```python
from build123d import *

# Parameters (mm, degrees)
F0_R        = 2.5
F1_DEPTH    = 3
F3_DEPTH    = 1
F4_T1_DEPTH = 1


# Not quite as in the source:
# - a fillet or chamfer that OpenCascade refuses, or shapes differently, is made with other operations: its cross-section is extruded or revolved along the edge and cut away or added


with BuildPart() as f1:
    # F0 (on Top) → F1 (new body)
    with BuildSketch(Plane.XY):
        with BuildLine():
            Line((42.1995138221, 67.0275468757), (33.4926469464, 67.1294207869))
            ThreePointArc((33.4926469464, 67.1294207869), (32.7404851321, 62.3046461892), (30.658157874, 57.8878475177))
            ThreePointArc((30.658157874, 57.8878475177), (27.294204133, 42.9798709067), (13.9152540739, 50.3668626301))
            ThreePointArc((13.9152540739, 50.3668626301), (12.375918121, 50.6607466073), (10.86986377, 51.0940170307))
            Line((10.86986377, 51.0940170307), (8.0824060906, 42.844775322))
            ThreePointArc((8.0824060906, 42.844775322), (12.4386086282, 40.6384895823), (15.9957592753, 37.2932128243))
            ThreePointArc((15.9957592753, 37.2932128243), (29.1345687017, 29.4870845738), (17.9747991522, 19.0456529188))
            ThreePointArc((17.9747991522, 19.0456529188), (17.2196179112, 17.6724725733), (16.3421568627, 16.3740176929))
            Line((16.3421568627, 16.3740176929), (23.3262801503, 11.1738320243))
            ThreePointArc((23.3262801503, 11.1738320243), (26.7707231948, 14.6350470461), (31.0514904559, 16.9843509793))
            ThreePointArc((31.0514904559, 16.9843509793), (42.5356749941, 27.0678750109), (49.017508165, 13.2277236335))
            ThreePointArc((49.017508165, 13.2277236335), (50.0901164433, 12.0851675302), (51.0538700425, 10.8494078578))
            Line((51.0538700425, 10.8494078578), (58.1577532953, 15.8847580755))
            ThreePointArc((58.1577532953, 15.8847580755), (55.9303336315, 20.230192341), (55.0188426496, 25.0274187796))
            ThreePointArc((55.0188426496, 25.0274187796), (48.977649601, 39.065507608), (64.1434123595, 40.9532553024))
            ThreePointArc((64.1434123595, 40.9532553024), (65.5615019731, 41.620297142), (67.0345955027, 42.1550105429))
            Line((67.0345955027, 42.1550105429), (64.4409135174, 50.4672137913))
            ThreePointArc((64.4409135174, 50.4672137913), (59.6198494134, 49.6916248415), (54.7757497452, 50.307169899))
            ThreePointArc((54.7757497452, 50.307169899), (39.5579025703, 48.8996619005), (42.4490262494, 63.9065055152))
            ThreePointArc((42.4490262494, 63.9065055152), (42.2528455514, 65.4613161473), (42.1995138221, 67.0275468757))
        make_face()
        with Locations((37.5, 37.5)):
            Circle(F0_R, mode=Mode.SUBTRACT)
    extrude(amount=F1_DEPTH)

    # F2 (on face) → F3 (cut)
    with BuildSketch(Plane.XY.offset(3)):
        Polygon((40.25, 67.1147092408), (34.75, 67.1147092408), (40.25, 67.0503569865), align=None)
        with BuildLine():
            Line((31.7569283434, 42.2575582148), (28.1635644564, 43.4251129174))
            ThreePointArc((28.1635644564, 43.4251129174), (20.4254111601, 42.6084822131), (14.6451171229, 47.8175227185))
            Line((14.6451171229, 47.8175227185), (10.2457371637, 49.2469679185))
            Line((10.2457371637, 49.2469679185), (8.4849410638, 44.0360430191))
            Line((8.4849410638, 44.0360430191), (30.0573348743, 37.0267473751))
            Line((30.0573348743, 37.0267473751), (31.7569283434, 42.2575582148))
        make_face()
        with BuildLine():
            Line((31.2005865164, 33.5081806175), (28.9797655003, 30.4514827223))
            ThreePointArc((28.9797655003, 30.4514827223), (27.3652065793, 22.8397088401), (20.6249055731, 18.9520045705))
            Line((20.6249055731, 18.9520045705), (17.9059392288, 15.2096684519))
            Line((17.9059392288, 15.2096684519), (22.3177073919, 11.9247874969))
            Line((22.3177073919, 11.9247874969), (35.6501799855, 30.2753617299))
            Line((35.6501799855, 30.2753617299), (31.2005865164, 33.5081806175))
        make_face()
        with BuildLine():
            Line((52.6444673021, 11.9768495643), (57.1318860772, 15.1576063845))
            Line((57.1318860772, 15.1576063845), (43.7994134836, 33.5081806175))
            Line((43.7994134836, 33.5081806175), (39.3498200145, 30.2753617299))
            Line((39.3498200145, 30.2753617299), (41.5706410307, 27.2186638347))
            ThreePointArc((41.5706410307, 27.2186638347), (48.3109420369, 23.3309595651), (49.9255009579, 15.7191856828))
            Line((49.9255009579, 15.7191856828), (52.6444673021, 11.9768495643))
        make_face()
        with BuildLine():
            Line((66.4538563054, 44.0161570789), (64.8154654671, 49.2668538587))
            Line((64.8154654671, 49.2668538587), (43.2430716566, 42.2575582148))
            Line((43.2430716566, 42.2575582148), (44.9426651257, 37.0267473751))
            Line((44.9426651257, 37.0267473751), (48.5360290127, 38.1943020778))
            ThreePointArc((48.5360290127, 38.1943020778), (54.3163230499, 43.4033425831), (62.0544763461, 42.5867118789))
            Line((62.0544763461, 42.5867118789), (66.4538563054, 44.0161570789))
        make_face()
        with BuildLine():
            Line((34.75, 44.4321520627), (37.5, 44.4321520627))
            Line((37.5, 44.4321520627), (40.25, 44.4321520627))
            Line((40.25, 44.4321520627), (40.25, 48.2104384478))
            ThreePointArc((40.25, 48.2104384478), (37.0821171737, 55.3175067985), (40.25, 62.4245751493))
            Line((40.25, 62.4245751493), (40.25, 67.0503569865))
            Line((40.25, 67.0503569865), (34.75, 67.1147092408))
            Line((34.75, 67.1147092408), (34.75, 44.4321520627))
        make_face()
    extrude(amount=-F3_DEPTH, mode=Mode.SUBTRACT)

    # F4: fillet of radius 3 on 10 edges, made by hand

    # F4_s2 → F4_t1 (join)
    with BuildSketch(Plane.XY.offset(2)):
        with BuildLine():
            ThreePointArc((37.25, 44.4321520627), (39.3713203436, 45.3108317191), (40.25, 47.4321520627))
            Line((40.25, 47.4321520627), (40.25, 44.4321520627))
            Line((40.25, 44.4321520627), (37.25, 44.4321520627))
        make_face()
        with BuildLine():
            ThreePointArc((34.75, 47.4321520627), (35.6286796564, 45.3108317191), (37.75, 44.4321520627))
            Line((37.75, 44.4321520627), (34.75, 44.4321520627))
            Line((34.75, 44.4321520627), (34.75, 47.4321520627))
        make_face()
        with BuildLine():
            ThreePointArc((30.8298773603, 39.4043886659), (30.6497273839, 41.6934111482), (28.9037587945, 43.1846091979))
            Line((28.9037587945, 43.1846091979), (31.7569283434, 42.2575582148))
            Line((31.7569283434, 42.2575582148), (30.8298773603, 39.4043886659))
        make_face()
        with BuildLine():
            ThreePointArc((27.2041653254, 37.9537983583), (29.4931878078, 38.1339483346), (30.9843858575, 39.879916924))
            Line((30.9843858575, 39.879916924), (30.0573348743, 37.0267473751))
            Line((30.0573348743, 37.0267473751), (27.2041653254, 37.9537983583))
        make_face()
        with BuildLine():
            ThreePointArc((33.6276374995, 31.7448248606), (31.3949783475, 32.2808388993), (29.4372307595, 31.0811296344))
            Line((29.4372307595, 31.0811296344), (31.2005865164, 33.5081806175))
            Line((31.2005865164, 33.5081806175), (33.6276374995, 31.7448248606))
        make_face()
        with BuildLine():
            ThreePointArc((33.8868242286, 27.8483107468), (34.4228382672, 30.0809698988), (33.2231290023, 32.0387174868))
            Line((33.2231290023, 32.0387174868), (35.6501799855, 30.2753617299))
            Line((35.6501799855, 30.2753617299), (33.8868242286, 27.8483107468))
        make_face()
        with BuildLine():
            ThreePointArc((41.1131757714, 27.8483107468), (40.5771617328, 30.0809698988), (41.7768709977, 32.0387174868))
            Line((41.7768709977, 32.0387174868), (39.3498200145, 30.2753617299))
            Line((39.3498200145, 30.2753617299), (41.1131757714, 27.8483107468))
        make_face()
        with BuildLine():
            ThreePointArc((45.5627692405, 31.0811296344), (43.6050216525, 32.2808388993), (41.3723625005, 31.7448248606))
            Line((41.3723625005, 31.7448248606), (43.7994134836, 33.5081806175))
            Line((43.7994134836, 33.5081806175), (45.5627692405, 31.0811296344))
        make_face()
        with BuildLine():
            ThreePointArc((44.0156141425, 39.879916924), (45.5068121922, 38.1339483346), (47.7958346746, 37.9537983583))
            Line((47.7958346746, 37.9537983583), (44.9426651257, 37.0267473751))
            Line((44.9426651257, 37.0267473751), (44.0156141425, 39.879916924))
        make_face()
        with BuildLine():
            ThreePointArc((46.0962412055, 43.1846091979), (44.3502726161, 41.6934111482), (44.1701226397, 39.4043886659))
            Line((44.1701226397, 39.4043886659), (43.2430716566, 42.2575582148))
            Line((43.2430716566, 42.2575582148), (46.0962412055, 43.1846091979))
        make_face()
    extrude(amount=F4_T1_DEPTH)


solid = f1.part
```
Source: CAD feature listing. Evaluate the final solid. Frame: model axes, mm. A direction names the side the tool comes from. Round coordinates to 2 decimals unless told otherwise and drop trailing zeros. Loops run counter-clockwise (first coordinate to the right, second up) from the corner with the lowest first, then second, coordinate; pieces in that order, holes last. Notation, with made-up numbers: M 80,51.25 L 117,51.25 A26 cw 117,76.25 Z; hole C -1,15 d5. An arc over 180 degrees is marked long. Use a Markdown table: item, result. Add a question column.
1. Ray query, line 1 along X through (y, z) = (63, 2.2); line 2 along Z through (x, y) = (24.5, 39.5); line 3 along X through (y, z) = (47, 1.9). Return the intervals inside material, ascending. Write a range as [from, to].
2. Set-up query: faces 1 (the flat face through (12.48, 48.52, 2.51)), 2 (the cylindrical face through (17.23, 17.69, 1.48)), 3 (the flat face through (19.284, 17.107, 2.507)). Return all of +Z, -Z, +X, -X, +Y, -Y with unobstructed straight access to the full face (end or side cutting, diameter ignored); none if empty.
3. Contact query for flat-ended pins moving along their axis: pin 1 (1.6 mm diameter, centred on x = 37, y = 52.5, fed in from +Z); pin 2 (1.5 mm diameter, centred on y = 31.5, z = 1, fed in from -X); pin 3 (0.5 mm diameter, centred on y = 65, z = 2.5, fed in from -X). Output: stop coordinate, or through.
4. Cut plane C-C, the plane x = 19. Output: boundary loops of the cut face in (y, z), and give its area (3 significant figures).
5. Cut plane D-D, the plane y = 56.5. Output: boundary loops of the cut face in (x, z).
6. Cut plane B-B, the plane z = 1.45. Output: boundary loops of the cut face in (x, y), and give its area (3 significant figures).
7. Cut plane A-A, the plane y = 36. Output: boundary loops of the cut face in (x, z), and give its area (3 significant figures).
8. Pull-direction query (Y, two-part tool) for faces 4 (the cylindrical face through (35.521, 45.424, 2.493)), 5 (the cylindrical face through (65.54, 41.61, 1.48)), 6 (the cylindrical face through (48.86, 38.85, 1.15)); classes: +Y half, -Y half, draft (parallel to the pull), parting line (faces both ways), or undercut.
Solution:
| question | item | result |
|---|---|---|
| 1 | line 1 | x = [32.94, 34.75], [40.25, 40.95] |
| 1 | line 2 | z = [0, 2] |
| 1 | line 3 | x = [9.49, 15.06], [31.7, 41.93], [51.34, 65.52] |
| 2 | face 1 | +Z, -X |
| 2 | face 2 | +Z, -Z, -X |
| 2 | face 3 | +Z, -Y |
| 3 | pin 1 | stops at z = 2 |
| 3 | pin 2 | stops at x = 28.41 |
| 3 | pin 3 | stops at x = 33.3 |
| 4 | outline | M 14.4,0 L 18.92,0 L 18.92,3 L 16.72,3 L 16.72,2 L 14.4,2 Z; M 37.99,0 L 43.2,0 L 43.2,2 L 40.62,2 L 40.62,3 L 37.99,3 Z |
| 4 | area | 24.3 mm2 |
| 5 | outline | M 31.64,0 L 37.16,0 L 37.16,2 L 34.75,2 L 34.75,3 L 31.64,3 Z |
| 6 | outline | M 8.08,42.84 A17.14 cw 16,37.29 A9.56 cw long 17.97,19.05 A17.14 cw 16.34,16.37 L 23.33,11.17 A17.14 cw 31.05,16.98 A9.56 cw long 49.02,13.23 A17.14 cw 51.05,10.85 L 58.16,15.88 A17.14 cw 55.02,25.03 A9.56 cw long 64.14,40.95 A17.14 cw 67.03,42.16 L 64.44,50.47 A17.14 cw 54.78,50.31 A9.56 cw long 42.45,63.91 A17.14 cw 42.2,67.03 L 33.49,67.13 A17.14 cw 30.66,57.89 A9.56 cw long 13.92,50.37 A17.14 cw 10.87,51.09 Z; hole C 37.5,37.5 d5 |
| 6 | area | 972 mm2 |
| 7 | outline | M 25.5,0 L 35.5,0 L 35.5,3 L 25.5,3 Z; M 39.5,0 L 47.86,0 L 47.86,3 L 39.5,3 Z |
| 7 | area | 55.1 mm2 |
| 8 | face 4 | +Y half |
| 8 | face 5 | -Y half |
| 8 | face 6 | undercut |
